```python
from build123d import *

# Parameters (mm, degrees)
SKETCH1_W           = 25
SKETCH1_H           = 24
SKETCH1_R           = 1.05
BOSS_EXTRUDE1_DEPTH = 1
SKETCH2_W           = 20.8
SKETCH2_H           = 5.5
BOSS_EXTRUDE2_DEPTH = 2.4
SKETCH3_W           = 8
SKETCH3_H           = 8
BOSS_EXTRUDE3_DEPTH = 4.9
CUT_EXTRUDE3_DEPTH  = 2
SKETCH7_R           = 2.038197989
SKETCH7_R_2         = 1.367783091
CUT_EXTRUDE4_DEPTH  = 0.5
SKETCH8_W           = 6
SKETCH8_H           = 2.224607268
BOSS_EXTRUDE4_DEPTH = 1


with BuildPart() as part:
    # Sketch1 → Boss-Extrude1 (new body)
    with BuildSketch(Plane.XY):
        Rectangle(SKETCH1_W, SKETCH1_H)
        with Locations((-10.5, 2.5)):
            Circle(SKETCH1_R, mode=Mode.SUBTRACT)
        with Locations((-10.5, -10)):
            Circle(SKETCH1_R, mode=Mode.SUBTRACT)
        with Locations((10.5, -10)):
            Circle(SKETCH1_R, mode=Mode.SUBTRACT)
        with Locations((10.5, 2.5)):
            Circle(SKETCH1_R, mode=Mode.SUBTRACT)
    extrude(amount=BOSS_EXTRUDE1_DEPTH)

    # Sketch2 → Boss-Extrude2 (add)
    with BuildSketch(Plane(origin=(0, 0, 0), x_dir=(-1, 0, 0), z_dir=(0, 0, -1))):
        with Locations((0, 9.25)):
            Rectangle(SKETCH2_W, SKETCH2_H)
    extrude(amount=BOSS_EXTRUDE2_DEPTH)

    # Sketch3 → Boss-Extrude3 (add)
    with BuildSketch(Plane.XY.offset(1)):
        with Locations((0, 2.5)):
            Rectangle(SKETCH3_W, SKETCH3_H)
    extrude(amount=BOSS_EXTRUDE3_DEPTH)

    # Sketch6 → Cut-Extrude3 (cut)
    with BuildSketch(Plane.XY.offset(5.9)):
        with BuildLine():
            Line((-4, 6.5), (-4, 2.499999997))
            ThreePointArc((-4, 2.499999997), (-2.828427126, 5.328427124), (0, 6.5))
            Line((0, 6.5), (-4, 6.5))
        make_face()
        with BuildLine():
            ThreePointArc((0, 6.5), (2.828427125, 5.328427125), (4, 2.5))
            Line((4, 2.5), (4, 6.5))
            Line((4, 6.5), (0, 6.5))
        make_face()
        with BuildLine():
            ThreePointArc((4, 2.5), (2.828427125, -0.328427125), (0, -1.5))
            Line((0, -1.5), (4, -1.5))
            Line((4, -1.5), (4, 2.5))
        make_face()
        with BuildLine():
            Line((-4, 2.499999997), (-4, -1.5))
            Line((-4, -1.5), (0, -1.5))
            ThreePointArc((0, -1.5), (-2.828427124, -0.328427126), (-4, 2.499999997))
        make_face()
    extrude(amount=-CUT_EXTRUDE3_DEPTH, mode=Mode.SUBTRACT)

    # Sketch7 → Cut-Extrude4 (cut)
    with BuildSketch(Plane.XY.offset(5.9)):
        with Locations((0, 2.5)):
            Circle(SKETCH7_R)
        with Locations((0, 2.5)):
            Circle(SKETCH7_R_2, mode=Mode.SUBTRACT)
    extrude(amount=-CUT_EXTRUDE4_DEPTH, mode=Mode.SUBTRACT)

    # Sketch8 → Boss-Extrude4 (add)
    with BuildSketch(Plane.XY.offset(1)):
        with Locations((0, -8.887696366)):
            Rectangle(SKETCH8_W, SKETCH8_H)
    extrude(amount=BOSS_EXTRUDE4_DEPTH)


solid = part.part
```
Part model, mm, in its own coordinate system. A direction names the side the tool comes from. Coordinates: 2 decimals unless noted, no trailing zeros. Write each loop counter-clockwise with the first axis right and the second up, starting at its lowest first coordinate (ties: lowest second). Pieces come first, ordered by that corner, then holes.
Item 1: Slice it at D-D (x = 1.75). Write the cut outline in (y, z), and give its area (3 significant figures).
Item 2: Mould opens along Y. For faces 1 (the face through (0, -10, 1.5)), 2 (the face through (-4, 2, 2)), 3 (the face through (-9.94, -9.11, 0.49)) say: released by +Y, released by -Y, zero draft, split by the parting line, or undercut.
Item 3: Slice it at C-C (y = -8.25). Write the cut outline in (x, z), and give its area (3 significant figures).
Item 4: Which spindle directions (+Z, -Z, +X, -X, +Y, -Y) get a long thin tool onto all of the face, cutting with end or side? Do faces 4 (the face through (-3, -1, 3.9)), 5 (the face through (3, -1, 3.9)), 6 (the face through (4, 2, 2)), 7 (the face through (0, -2, 1)), 8 (the face through (0, -9, 2)). Say none if no direction does.
Item 5: Probe line 1 (Y direction, x = -10.5, z = 0.4); line 2 (Y direction, x = -1.25, z = 1.75); line 3 (Z direction, x = -10.25, y = -0.25). List the from-to ranges inside material, lowest first.
Item 6: Pin check, flat tips, straight feed: pin 1 (4 mm diameter, centred on y = 4, z = 3.5, fed in from +X); pin 2 (1.5 mm diameter, centred on x = -1, z = 3, fed in from -Y); pin 3 (4.5 mm diameter, centred on x = 0, y = 2.5, fed in from -Z); pin 4 (1.9 mm diameter, centred on x = -10.5, y = 2.5, fed in from -Z). Stop position of each tip, or through.
Item 7: Slice it at B-B (z = 0.5). Write the cut outline in (x, y), and give its area (3 significant figures).
Item 8: Slice it at A-A (y = 1.75). Write the cut outline in (x, z), and give its area (3 significant figures).
Results found:
1. outline: (-12, 0) - (6.5, 0) - (6.5, -2.4) - (12, -2.4) - (12, 1) - (6.5, 1) - (6.5, 3.9) - (6.1, 3.9) - (6.1, 5.9) - (3.54, 5.9) - (3.54, 5.4) - (1.46, 5.4) - (1.46, 5.9) - (-1.1, 5.9) - (-1.1, 3.9) - (-1.5, 3.9) - (-1.5, 1) - (-7.78, 1) - (-7.78, 2) - (-10, 2) - (-10, 1) - (-12, 1) - close
1. area: 76.0 mm2
2. face 1: released by -Y
2. face 2: zero draft
2. face 3: undercut
3. outline: (-12.5, 0) - (12.5, 0) - (12.5, 1) - (3, 1) - (3, 2) - (-3, 2) - (-3, 1) - (-12.5, 1) - close
3. area: 31.0 mm2
4. face 4: +Z, -X, -Y
4. face 5: +Z, +X, -Y
4. face 6: +Z, +X, +Y, -Y
4. face 7: +Z
4. face 8: +Z, +X, -X, -Y
5. line 1: y = -12 to -11.05, -8.95 to 1.45, 3.55 to 12
5. line 2: y = -10 to -7.78, -1.5 to 6.5
5. line 3: z = 0 to 1
6. pin 1: stops at x = 4
6. pin 2: stops at y = -1.5
6. pin 3: stops at z = 0
6. pin 4: passes through
7. outline: (-12.5, -12) - (12.5, -12) - (12.5, 12) - (-12.5, 12) - close; hole circle Ø2.1 at (-10.5, -10); hole circle Ø2.1 at (-10.5, 2.5); hole circle Ø2.1 at (10.5, -10); hole circle Ø2.1 at (10.5, 2.5)
7. area: 586 mm2
8. outline: (-12.5, 0) - (-11.23, 0) - (-11.23, 1) - (-12.5, 1) - close; (-9.77, 0) - (9.77, 0) - (9.77, 1) - (4, 1) - (4, 3.9) - (3.93, 3.9) - (3.93, 5.9) - (1.9, 5.9) - (1.9, 5.4) - (1.14, 5.4) - (1.14, 5.9) - (-1.14, 5.9) - (-1.14, 5.4) - (-1.9, 5.4) - (-1.9, 5.9) - (-3.93, 5.9) - (-3.93, 3.9) - (-4, 3.9) - (-4, 1) - (-9.77, 1) - close; (11.23, 0) - (12.5, 0) - (12.5, 1) - (11.23, 1) - close
8. area: 60.2 mm2
